Could you check a few things on this drawing? It's one solid part, dimensions in mm from its lowest x, y, z. A direction names the side the tool comes from. Give positions to 0.01 mm unless a question says otherwise; leave off trailing zeros. Order: outer loops, then holes, each group sorted by start corner. A loop starts at its lowest first (then second) coordinate and runs counter-clockwise, first axis right, second up. Notation, with made-up numbers: M 37,35.5 L 86,35.5 A21 ccw 86,39.5 Z; hole C -32,80 d5. An arc over 180 degrees is marked long. Use one line per item in the form item = value.
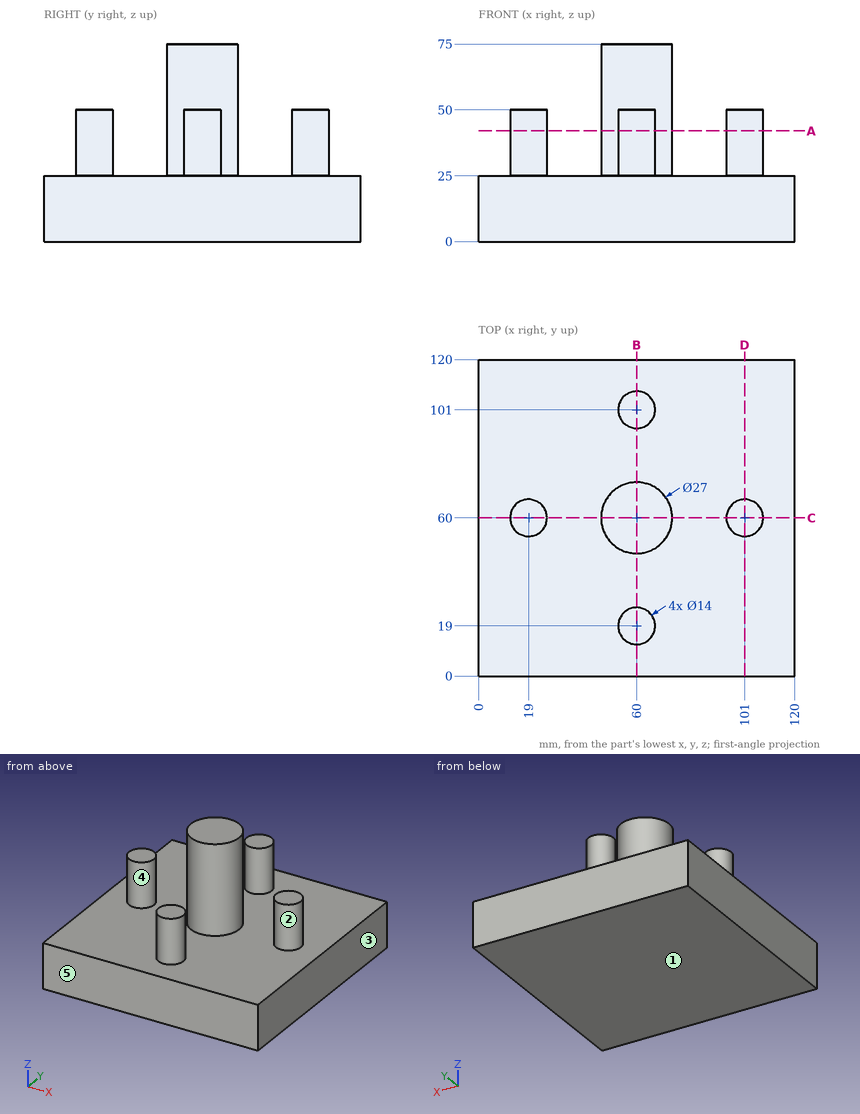
Q1. I want a section at A-A on z = 42. Write out the boundary of the cut face in (x, y).
Found:
outline = C 19,60 d14; C 60,60 d27; C 60,19 d14; C 60,101 d14; C 101,60 d14
Q2. I want a section at D-D on x = 101. Write out the boundary of the cut face in (y, z).
Found:
outline = M 0,0 L 120,0 L 120,25 L 67,25 L 67,50 L 53,50 L 53,25 L 0,25 Z
Q3. Thinking about a two-plate mould opening in X: for the marked faces 3, 4 and 5, which applies, +X half, -X half, draft (parallel to the pull), parting line (faces both ways), or undercut?
Found:
face_3 = +X half
face_4 = undercut
face_5 = draft
Q4. I'm going to push flat-ended pins straight in: pin 1 Ø6 at (x, y) = (25, 44.5) entering from +Z; pin 2 Ø4 at (x, y) = (63, 98.5) entering from +Z; pin 3 Ø8 at (x, z) = (21.5, 56.5) entering from +Y. Where does each tip first touch, or does it pass through?
Found:
pin_1 = 25
pin_2 = 50
pin_3 = through
Q5. On a 3-axis mill with a long thin cutter (end or side, diameter ignored), from which of +Z, -Z, +X, -X, +Y, -Y can I reach the whole of each face in a straight line? I mean the marked faces 1 and 2. Say none if no direction works.
Found:
face_1 = -Z, +X, -X, +Y, -Y
face_2 = +Z
Q6. I want a section at B-B on x = 60. Write out the boundary of the cut face in (y, z), then the cut area to 3 significant figures.
Found:
outline = M 0,0 L 120,0 L 120,25 L 108,25 L 108,50 L 94,50 L 94,25 L 73.5,25 L 73.5,75 L 46.5,75 L 46.5,25 L 26,25 L 26,50 L 12,50 L 12,25 L 0,25 Z
area = 5,050 mm²
Q7. I need wall thicknesses on L1, parallel to X at y = 63.5, z = 46; L2, parallel to Z at x = 94, y = 44; L3, parallel to Z at x = 96.5, y = 58. Which ranges of each line are inside material? Lowest first, please.
Found:
L1 = 12.94 to 25.06, 46.96 to 73.04, 94.94 to 107.06
L2 = 0 to 25
L3 = 0 to 50
